Check sheet for the drawn part. Datum: minimum x, y, z corner. Units: mm. Round coordinates to 2 decimals unless told otherwise and drop trailing zeros. Order: outer loops, then holes, each group sorted by start corner. A loop starts at its lowest first (then second) coordinate and runs counter-clockwise, first axis right, second up. Notation, with made-up numbers: M 69,59 L 103,59 A17 cw 103,80 Z; hole C -0.5,33.25 d4. An arc over 180 degrees is marked long. Answer as a JSON object with one key per item and string values. Group by question number.
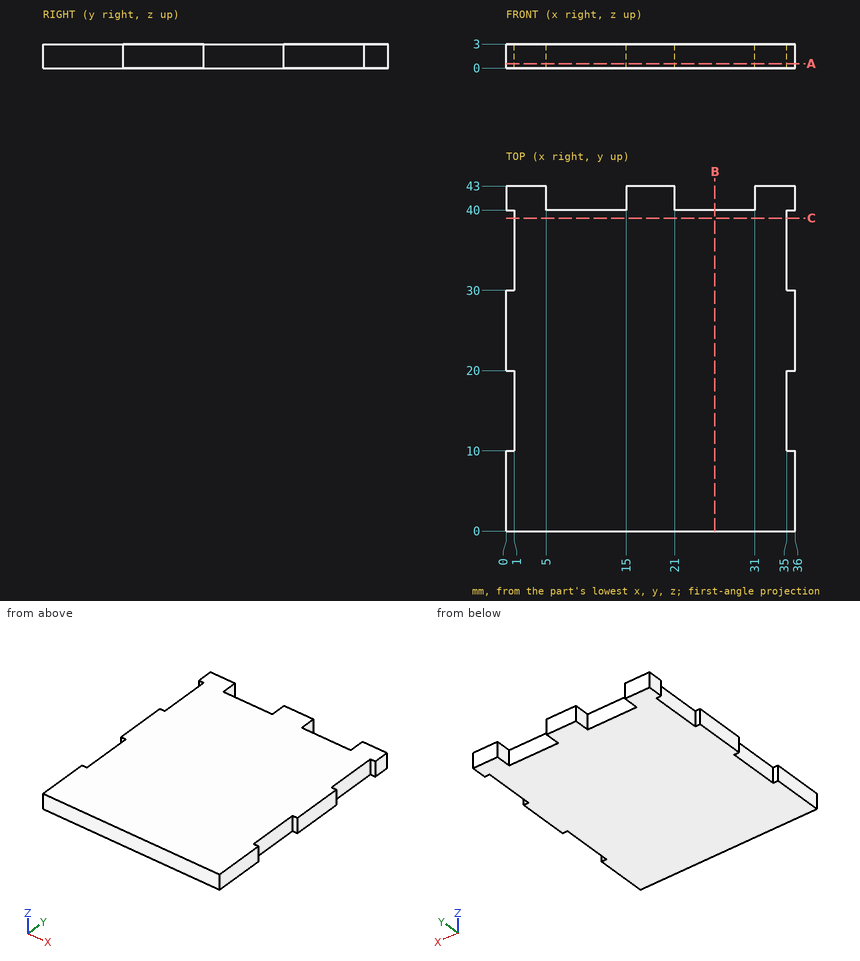
1) Go/stop test with flat-tipped pins: P1, Ø1.5, axis at y = 16.5, z = 2, coming from the -X side; P2, Ø0.9, axis at x = 26, z = 1, coming from the +Y side; P3, Ø1, axis at y = 16.5, z = 2, coming from the +X side. Record where each tip stops, or that it passes through.
2) Sectioned sample at A-A (z = 0.55). Record the boundary of the cut face in (x, y), then the cut area to 3 significant figures.
3) Thickness scan on line 1 along X through (y, z) = (41.5, 2.85); line 2 along Y through (x, z) = (12.5, 0.9); line 3 along X through (y, z) = (19, 2.85). Record the ranges inside material, lowest first. Write a range as [from, to].
4) Sectioned sample at B-B (x = 26). Record the boundary of the cut face in (y, z).
5) Sectioned sample at C-C (y = 39). Record the boundary of the cut face in (x, z), then the cut area to 3 significant figures.
Final values:
{
 "1": {"P1": "stops at x = 1", "P2": "stops at y = 40", "P3": "stops at x = 35"},
 "2": {"outline": "M 0,0 L 36,0 L 36,10 L 35,10 L 35,20 L 36,20 L 36,30 L 35,30 L 35,40 L 36,40 L 36,43 L 31,43 L 31,40 L 21,40 L 21,43 L 15,43 L 15,40 L 5,40 L 5,43 L 0,43 L 0,40 L 1,40 L 1,30 L 0,30 L 0,20 L 1,20 L 1,10 L 0,10 Z", "area": "1,450 mm^2"},
 "3": {"line 1": "x = [0, 5], [15, 21], [31, 36]", "line 2": "y = [0, 40]", "line 3": "x = [1, 35]"},
 "4": {"outline": "M 0,0 L 40,0 L 40,3 L 0,3 Z"},
 "5": {"outline": "M 1,0 L 35,0 L 35,3 L 1,3 Z", "area": "102 mm^2"}
}
